Could you check a few things on this model? Use its own coordinates, in mm. A direction names the side the tool comes from. Round coordinates to 2 decimals unless told otherwise and drop trailing zeros. Loops run counter-clockwise (first coordinate to the right, second up) from the corner with the lowest first, then second, coordinate; pieces in that order, holes last.
from build123d import *

# Parameters (mm, degrees)
F0_R      = 13.97
F1_DEPTH  = 12.7
F2_R      = 12.7
F3_DEPTH  = 12.7
F4_R      = 11.43
F5_DEPTH  = 12.7
F6_R      = 10.16
F7_DEPTH  = 12.7
F8_R      = 8.89
F9_DEPTH  = 12.7
F10_R     = 7.62
F11_DEPTH = 12.7
F12_R     = 6.35
F13_DEPTH = 12.7
F14_R     = 5.08
F15_DEPTH = 12.7
F16_R     = 3.81
F17_DEPTH = 12.7
F18_R     = 2.54
F19_DEPTH = 12.7
F20_R     = 1.274309
F21_DEPTH = 12.7


with BuildPart() as f1:
    # F0 (on Top) → F1 (new body)
    with BuildSketch(Plane.XY):
        Circle(F0_R)
    extrude(amount=F1_DEPTH)

    # F2 (on face) → F3 (join)
    with BuildSketch(Plane.XY.offset(12.7)):
        Circle(F2_R)
    extrude(amount=F3_DEPTH)

    # F4 (on face) → F5 (join)
    with BuildSketch(Plane.XY.offset(25.4)):
        Circle(F4_R)
    extrude(amount=F5_DEPTH)

    # F6 (on face) → F7 (join)
    with BuildSketch(Plane.XY.offset(38.1)):
        Circle(F6_R)
    extrude(amount=F7_DEPTH)

    # F8 (on face) → F9 (join)
    with BuildSketch(Plane.XY.offset(50.8)):
        Circle(F8_R)
    extrude(amount=F9_DEPTH)

    # F10 (on face) → F11 (join)
    with BuildSketch(Plane.XY.offset(63.5)):
        Circle(F10_R)
    extrude(amount=F11_DEPTH)

    # F12 (on face) → F13 (join)
    with BuildSketch(Plane.XY.offset(76.2)):
        Circle(F12_R)
    extrude(amount=F13_DEPTH)

    # F14 (on face) → F15 (join)
    with BuildSketch(Plane.XY.offset(88.9)):
        Circle(F14_R)
    extrude(amount=F15_DEPTH)

    # F16 (on face) → F17 (join)
    with BuildSketch(Plane.XY.offset(101.6)):
        Circle(F16_R)
    extrude(amount=F17_DEPTH)

    # F18 (on face) → F19 (join)
    with BuildSketch(Plane.XY.offset(114.3)):
        Circle(F18_R)
    extrude(amount=F19_DEPTH)

    # F20 (on face) → F21 (join)
    with BuildSketch(Plane.XY.offset(127)):
        Circle(F20_R)
    extrude(amount=F21_DEPTH)


solid = f1.part
Item 1: If we section it at B-B, the plane z = 23: Please give me the cut outline in (x, y), then the cut area to 3 significant figures.
Results list:
outline: circle Ø25.4 at (0, 0)
area: 507 mm2
Item 2: For faces 1 (the cylindrical face through (-0.83, -3.72, 107.86)), 2 (the flat face through (0, 0, 0)), which set-ups out of +Z, -Z, +X, -X, +Y, -Y let a thin tool reach every point of the face, with its end or its side?
Results list:
face 1: +Z
face 2: -Z, +X, -X, +Y, -Y
Item 3: Will these pins go through, and if not, where does the flat tip stop? pin 1 (10 mm diameter, centred on x = -2.5, y = -1, fed in from +Z); pin 2 (4.5 mm diameter, centred on x = 2.5, y = 3, fed in from +Z); pin 3 (12 mm diameter, centred on x = 8, z = 50.5, fed in from -Y); pin 4 (6 mm diameter, centred on y = -7.5, z = 29.5, fed in from -X).
Results list:
pin 1: stops at z = 139.7
pin 2: stops at z = 127
pin 3: stops at y = -9.96
pin 4: stops at x = -10.51
Item 4: If I drill on line 1 along Z through (x, y) = (-2.75, -6.75); line 2 along Z through (x, y) = (-1, -9.75); line 3 along X through (y, z) = (5.5, 19), over which ranges is the centre line in solid material (lowest first)?
Results list:
line 1: z = 0 to 76.2
line 2: z = 0 to 50.8
line 3: x = -11.45 to 11.45
Item 5: If we section it at A-A, the plane z = 41: Please give me the cut outline in (x, y), then the cut area to 3 significant figures.
Results list:
outline: circle Ø20.32 at (0, 0)
area: 324 mm2
